The figure shows three views and two pictorial views of one solid part (mm, origin at its lowest corner). Answer the questions. A direction names the side the tool comes from. Coordinates: 2 decimals unless noted, no trailing zeros. Loops run counter-clockwise (first coordinate to the right, second up) from the corner with the lowest first, then second, coordinate; pieces in that order, holes last.
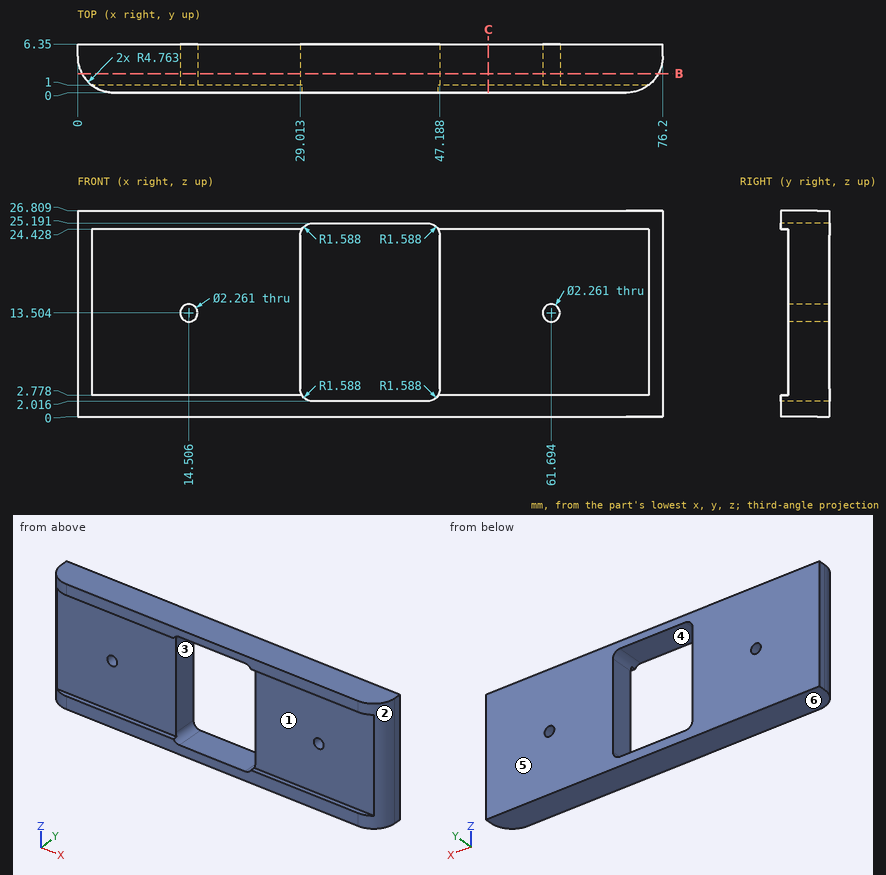
Q1. Flat-ended cylindrical pins translate along their axes: pin 1 Ø1.8 at (x, z) = (14.51, 13.5) entering from +Y; pin 2 Ø1 at (y, z) = (1.5, 16.5) entering from +X; pin 3 Ø1.5 at (y, z) = (1.5, 4.5) entering from -X. Find the tip coordinate at first contact, or state that the pin passes through.
Findings below:
pin 1: passes through
pin 2: stops at x = 75.32
pin 3: stops at x = 0.72
Q2. Which of the six approach directions +Z, -Z, +X, -X, +Y, -Y give full straight-line access (tool end or side, diameter ignored) to the marked faces 1, 2 and 3?
Findings below:
face 1: +X, -X, -Y
face 2: +Z, -Z, +X, -Y
face 3: +Y, -Y
Q3. A cutting plane is placed at C-C (x = 53.5). Give the vertices of the cut face in (y, z).
Findings below:
outline: (0, 0) - (6.35, 0) - (6.35, 26.81) - (0, 26.81) - (0, 24.43) - (1, 24.43) - (1, 2.78) - (0, 2.78) - close
Q4. Determine the mould class of the marked faces 4, 5 and 6 for opening direction Z: +Z half, -Z half, draft (parallel to the pull), parting line (faces both ways), or undercut.
Findings below:
face 4: undercut
face 5: draft
face 6: -Z half
Q5. Straight lines are drawn through the part: probe 1 along X at (y, z) = (5, 10.5); probe 2 along Z at (x, y) = (39.5, 2.25) (1 decimal); probe 3 along Y at (x, z) = (58, 16). For each, find the intervals that lie inside material, in ascending order.
Findings below:
probe 1: x = 0 to 29.01, 47.19 to 76.2
probe 2: z = 0 to 2, 25.2 to 26.8
probe 3: y = 1 to 6.35
Q6. A cutting plane is placed at B-B (y = 2.5). Give the vertices of the cut face in (x, z) (1 decimal).
Findings below:
outline: (0.6, 0) - (75.6, 0) - (75.6, 26.8) - (0.6, 26.8) - close; hole circle Ø2.3 at (14.5, 13.5); hole (29, 3.6) arc R1.6 ccw to (30.6, 2) - (45.6, 2) arc R1.6 ccw to (47.2, 3.6) - (47.2, 23.6) arc R1.6 ccw to (45.6, 25.2) - (30.6, 25.2) arc R1.6 ccw to (29, 23.6) - close; hole circle Ø2.3 at (61.7, 13.5)
